The listing builds one solid part. Answer for the finished solid, in the listing's coordinates (mm). A direction names the side the tool comes from. Coordinates: 2 decimals unless noted, no trailing zeros. Write each loop counter-clockwise with the first axis right and the second up, starting at its lowest first coordinate (ties: lowest second). Pieces come first, ordered by that corner, then holes.
from build123d import *

# Parameters (mm, degrees)
F0_R     = 6
F0_R_2   = 2.5
F1_DEPTH = 5
F3_DEPTH = 25
F4_R     = 2.35
F5_DEPTH = 3
F6_R     = 1
F7_DEPTH = 25


with BuildPart() as f1:
    # F0 (on Top) → F1 (new body)
    with BuildSketch(Plane.XY):
        Circle(F0_R)
        Circle(F0_R_2, mode=Mode.SUBTRACT)
        Circle(F0_R_2)
    extrude(amount=F1_DEPTH)

    # F2 (on face) → F3 (cut)
    with BuildSketch(Plane(origin=(0, 0, 0), x_dir=(1, 0, 0), z_dir=(0, 0, -1))):
        with BuildLine():
            ThreePointArc((-0.5161768662, 3.4617281006), (0, 3.5), (0.5161768662, 3.4617281006))
            Line((0.5161768662, 3.4617281006), (1.5986529108, 5.7831054695))
            ThreePointArc((1.5986529108, 5.7831054695), (0, 6), (-1.5986529108, 5.7831054695))
            Line((-1.5986529108, 5.7831054695), (-0.5161768662, 3.4617281006))
        make_face()
        with BuildLine():
            ThreePointArc((-2.4523485819, 2.4971957138), (-2.057248383, 2.8315594803), (-1.6171568681, 3.1039980129))
            Line((-1.6171568681, 3.1039980129), (-2.1058867345, 5.6182952095))
            ThreePointArc((-2.1058867345, 5.6182952095), (-3.5267115138, 4.8541019662), (-4.6925614803, 3.7389660006))
            Line((-4.6925614803, 3.7389660006), (-2.4523485819, 2.4971957138))
        make_face()
        with BuildLine():
            ThreePointArc((-3.4518064915, 0.5788194408), (-3.328697807, 1.0815594803), (-3.132791644, 1.5606461852))
            Line((-3.132791644, 1.5606461852), (-5.0060492236, 3.3074871384))
            ThreePointArc((-5.0060492236, 3.3074871384), (-5.7063390978, 1.8541019662), (-5.9940710587, 0.2666686023))
            Line((-5.9940710587, 0.2666686023), (-3.4518064915, 0.5788194408))
        make_face()
        with BuildLine():
            Line((-5.0060492236, -3.3074871384), (-3.132791644, -1.5606461852))
            ThreePointArc((-3.132791644, -1.5606461852), (-3.328697807, -1.0815594803), (-3.4518064915, -0.5788194408))
            Line((-3.4518064915, -0.5788194408), (-5.9940710587, -0.2666686023))
            ThreePointArc((-5.9940710587, -0.2666686023), (-5.7063390978, -1.8541019662), (-5.0060492236, -3.3074871384))
        make_face()
        with BuildLine():
            Line((-2.1058867345, -5.6182952095), (-1.6171568681, -3.1039980129))
            ThreePointArc((-1.6171568681, -3.1039980129), (-2.057248383, -2.8315594803), (-2.4523485819, -2.4971957138))
            Line((-2.4523485819, -2.4971957138), (-4.6925614803, -3.7389660006))
            ThreePointArc((-4.6925614803, -3.7389660006), (-3.5267115138, -4.8541019662), (-2.1058867345, -5.6182952095))
        make_face()
        with BuildLine():
            Line((1.5986529108, -5.7831054695), (0.5161768662, -3.4617281006))
            ThreePointArc((0.5161768662, -3.4617281006), (0, -3.5), (-0.5161768662, -3.4617281006))
            Line((-0.5161768662, -3.4617281006), (-1.5986529108, -5.7831054695))
            ThreePointArc((-1.5986529108, -5.7831054695), (0, -6), (1.5986529108, -5.7831054695))
        make_face()
        with BuildLine():
            Line((4.6925614803, -3.7389660006), (2.4523485819, -2.4971957138))
            ThreePointArc((2.4523485819, -2.4971957138), (2.057248383, -2.8315594803), (1.6171568681, -3.1039980129))
            Line((1.6171568681, -3.1039980129), (2.1058867345, -5.6182952095))
            ThreePointArc((2.1058867345, -5.6182952095), (3.5267115138, -4.8541019662), (4.6925614803, -3.7389660006))
        make_face()
        with BuildLine():
            Line((5.9940710587, -0.2666686023), (3.4518064915, -0.5788194408))
            ThreePointArc((3.4518064915, -0.5788194408), (3.328697807, -1.0815594803), (3.132791644, -1.5606461852))
            Line((3.132791644, -1.5606461852), (5.0060492236, -3.3074871384))
            ThreePointArc((5.0060492236, -3.3074871384), (5.7063390978, -1.8541019662), (5.9940710587, -0.2666686023))
        make_face()
        with BuildLine():
            ThreePointArc((3.132791644, 1.5606461852), (3.328697807, 1.0815594803), (3.4518064915, 0.5788194408))
            Line((3.4518064915, 0.5788194408), (5.9940710587, 0.2666686023))
            ThreePointArc((5.9940710587, 0.2666686023), (5.7063390978, 1.8541019662), (5.0060492236, 3.3074871384))
            Line((5.0060492236, 3.3074871384), (3.132791644, 1.5606461852))
        make_face()
        with BuildLine():
            ThreePointArc((1.6171568681, 3.1039980129), (2.057248383, 2.8315594803), (2.4523485819, 2.4971957138))
            Line((2.4523485819, 2.4971957138), (4.6925614803, 3.7389660006))
            ThreePointArc((4.6925614803, 3.7389660006), (3.5267115138, 4.8541019662), (2.1058867345, 5.6182952095))
            Line((2.1058867345, 5.6182952095), (1.6171568681, 3.1039980129))
        make_face()
    extrude(amount=-F3_DEPTH, mode=Mode.SUBTRACT)

    # F4 (on face) → F5 (cut)
    with BuildSketch(Plane(origin=(0, 0, 0), x_dir=(1, 0, 0), z_dir=(0, 0, -1))):
        Circle(F4_R)
    extrude(amount=-F5_DEPTH, mode=Mode.SUBTRACT)

    # F6 (on face) → F7 (cut)
    with BuildSketch(Plane(origin=(0, 0, 0), x_dir=(1, 0, 0), z_dir=(0, 0, -1))):
        Circle(F6_R)
    extrude(amount=-F7_DEPTH, mode=Mode.SUBTRACT)


solid = f1.part
Q1. Determine the mould class of faces 1 (the face through (-1.4, 0.1, 5)), 2 (the face through (3.56, -3.11, 2.46)), 3 (the face through (-4.083, 2.446, 2.465)) for opening direction Y: released by +Y, released by -Y, zero draft, split by the parting line, or undercut.
Answers below:
face 1: zero draft
face 2: released by -Y
face 3: undercut
Q2. Which of the six approach directions +Z, -Z, +X, -X, +Y, -Y give full straight-line access (tool end or side, diameter ignored) to faces 4 (the face through (-2.1, -2.8, 2.5)), 5 (the face through (3.331, 1.075, 2.465)), 6 (the face through (1.05, -4.61, 2.46)), 7 (the face through (-0.509, 2.294, 1.479))?
Answers below:
face 4: +Z, -Z
face 5: +Z, -Z, +X
face 6: +Z, -Z, -Y
face 7: -Z
Q3. The part is cut by section A-A, the plane y = 0. Write down the section's boundary in (x, z), then the cut area to 3 significant figures.
Answers below:
outline: (-6, 0) - (-2.35, 0) - (-2.35, 3) - (-1, 3) - (-1, 5) - (-6, 5) - close; (1, 3) - (2.35, 3) - (2.35, 0) - (6, 0) - (6, 5) - (1, 5) - close
area: 41.9 mm2
Q4. Find the intervals of material crossed by probe 1 along X at (y, z) = (0, 2.45); probe 2 along Y at (x, z) = (0, 1.7); probe 3 along Y at (x, z) = (4.25, 1.7), in increasing order.
Answers below:
probe 1: x = -6 to -2.35, 2.35 to 6
probe 2: y = -3.5 to -2.35, 2.35 to 3.5
probe 3: y = -3.49 to -2.6, -0.48 to 0.48, 2.6 to 3.49
Q5. The part is cut by section D-D, the plane y = -1.75. Write down the section's boundary in (x, z).
Answers below:
outline: (-3.34, 0) - (-1.57, 0) - (-1.57, 3) - (1.57, 3) - (1.57, 0) - (3.34, 0) - (3.34, 5) - (-3.34, 5) - close
Q6. The part is cut by section B-B, the plane x = 0. Write down the section's boundary in (y, z).
Answers below:
outline: (-3.5, 0) - (-2.35, 0) - (-2.35, 3) - (-1, 3) - (-1, 5) - (-3.5, 5) - close; (1, 3) - (2.35, 3) - (2.35, 0) - (3.5, 0) - (3.5, 5) - (1, 5) - close
Q7. The part is cut by section C-C, the plane x = 4. Write down the section's boundary in (y, z), then the cut area to 3 significant figures.
Answers below:
outline: (-3.36, 0) - (-2.37, 0) - (-2.37, 5) - (-3.36, 5) - close; (-0.51, 0) - (0.51, 0) - (0.51, 5) - (-0.51, 5) - close; (2.37, 0) - (3.36, 0) - (3.36, 5) - (2.37, 5) - close
area: 15.0 mm2
Q8. Given pin 1 (1.2 mm diameter, centred on x = 0, y = 0, fed in from +Z); pin 2 (1.4 mm diameter, centred on x = 1, y = -1, fed in from -Z), each flat-ended and moving along its own axis, determine where each tip first touches the part or whether it passes through.
Answers below:
pin 1: passes through
pin 2: stops at z = 3
